Can you work these out from the model? Positions are in its coordinate system, mm. A direction names the side the tool comes from. Give positions to 0.01 mm unless a question says otherwise; leave off trailing zeros. Order: outer loops, then holes, each group sorted by start corner. A loop starts at its lowest first (then second) coordinate and runs counter-clockwise, first axis right, second up. Notation, with made-up numbers: M -5,-15.75 L 48,-15.75 A24 cw 48,22.25 Z; hole C -32.75,58 d5. An arc over 180 degrees is marked long. One line per question, with ' | ' between items. Start each with the question number.
1) Thinking about a two-plate mould opening in Z: for faces 4 (the flat face through (31.4, 12.5, -8.2)), 5 (the cylindrical face through (181.574, 10.528, -7.396)), 6 (the flat face through (107.6, 11.5, -19.9)), 7 (the flat face through (109, 8.5, -4)), which applies, +Z half, -Z half, draft (parallel to the pull), parting line (faces both ways), or undercut?
2) I'm going to push flat-ended pins straight in: pin 1 Ø3 at (x, y) = (149.5, 12) entering from +Z; pin 2 Ø3.5 at (x, y) = (180.5, 17) entering from +Z; pin 3 Ø4.5 at (x, z) = (31.5, -7.5) entering from +Y; pin 4 Ø2 at (x, z) = (180, -6.9) entering from +Y. Where does each tip first touch, or does it pass through?
3) For faces 1 (the flat face through (180, 16, -9.8)), 2 (the cylindrical face through (28.69, 10.53, -5.9)), 3 (the flat face through (107, 18.5, -12)), which set-ups out of +Z, -Z, +X, -X, +Y, -Y let a thin tool reach every point of the face, with its end or its side?
4) If we section it at B-B, the plane z = -14: Please give me the cut outline in (x, y).
5) Please list where these lines run through material, in increasing order: line 1 along X through (y, z) = (9.65, -6.9); line 2 along X through (y, z) = (10.6, -6.9); line 3 along X through (y, z) = (14.5, -15). Write a range as [from, to].
6) If we section it at A-A, the plane x = 23.5: Please give me the cut outline in (y, z), plus the area to 3 significant figures.
Autodesk Inventor part; units mm, degrees
ref_plane "YZ Plane" through (0, 0, 0) normal (1, 0, 0) x (0, 1, 0)
ref_plane "XZ Plane" through (0, 0, 0) normal (0, 1, 0) x (-1, 0, 0)
ref_plane "XY Plane" through (0, 0, 0) normal (0, 0, 1) x (1, 0, 0)
sketch "Sketch1" plane through (0, 0, 0) normal (1, 0, 0) x (0, 1, 0)
  circle A0 centre (0, 0) radius 20
  line L0 (8.5, 8.5) -> (-16.9, 8.5)
  line L1 (8.5, 8.5) -> (8.5, -16.9)
  line L2 (0, 0) -> (0, 20)
  line L3 (0, 20) -> (-60.9241, 20)
  line L4 (-60.9241, 20) -> (-60.9241, 18.5)
  line L5 (-60.9241, 18.5) -> (0, 18.5)
  line L6 (0, 18.5) -> (0, 20)
  line L7 (0, 0) -> (14.1421, 14.1421)
  line L8 (0, 0) -> (20, 0)
  line L9 (-16.9, 8.5) -> (-16.9, 18.5)
  line L10 (-16.9, 8.5) -> (-22.9, 14.5)
  line L11 (-22.9, 14.5) -> (-22.9, 18.5)
  line L12 (12.3744, 12.3744) -> (12.1502, 13.2109)
  line L13 (11.3137, 13.435) -> (9.2071, 11.3284)
  line L14 (9.4313, 10.4919) -> (10.2678, 10.2678)
  line L15 (8.5, 8.5) -> (8.5, -16.9)
  line L16 (20, 0) -> (20, -60.9241)
  line L17 (20, -60.9241) -> (18.5, -60.9241)
  line L18 (18.5, -60.9241) -> (18.5, 0)
  line L19 (8.5, -16.9) -> (18.5, -16.9)
  line L20 (8.5, -16.9) -> (14.5, -22.9)
  line L21 (14.5, -22.9) -> (18.5, -22.9)
  arc A1 (9.2071, 11.3284) -> (9.4313, 10.4919) centre (9.5607, 10.9749) ccw
  arc A2 (12.1502, 13.2109) -> (11.3137, 13.435) centre (11.6673, 13.0815) ccw
  line L22 (10.4311, 10.4311) -> (9.483, 10.6851)
  arc A3 (9.3485, 11.187) -> (9.483, 10.6851) centre (9.5607, 10.9749) ccw
  line L23 (9.3485, 11.187) -> (11.4551, 13.2936)
  arc A4 (11.957, 13.1591) -> (11.4551, 13.2936) centre (11.6673, 13.0815) ccw
  line L24 (11.957, 13.1591) -> (12.2111, 12.2111)
  point P0 (0, 8.5)
  point P1 (-17.7041, 9.3041)
  point P2 (-16.9, 10.6953)
  point P3 (10.6953, -16.9)
  point P4 (9.3041, -17.7041)
  point P5 (18.5, 0)
  dimension "d0" = 40
  dimension "d1" = 25.4
  dimension "d2" = 1.5
  dimension "d4" = 45
  dimension "d6" = 45
  dimension "d7" = 4
  dimension "d8" = 10
  dimension "d10" = 2.5
  dimension "d11" = 2.5
  dimension "d12" = 60
  dimension "d13" = 1.5
  dimension "d15" = 0.5
  dimension "d16" = 0.2
extrude "Extrusion1" add sketch "Sketch1" along normal blind 216 contours L8 L1 L7 A0 | L18 L19 A0 | A0 L19 L1 L8 L18 | L19 L18 L21 L20 A0 | A0 L20 L19
sketch "Sketch3" plane through (0, 18.5, 0) normal (0, 1, 0) x (1, 0, 0)
  line L0 (0, 22.9) -> (0, 0)
  line L1 (0, 0) -> (216, 0)
  line L2 (216, 22.9) -> (216, 0)
  line L3 (0, 22.9) -> (216, 22.9)
  line L4 (0, 16.9) -> (216, 16.9)
  line L5 (28.3257, 4) -> (26.6514, 6.9)
  line L6 (26.6514, 6.9) -> (28.3257, 9.8)
  line L7 (28.3257, 9.8) -> (31.6743, 9.8)
  line L8 (31.6743, 9.8) -> (33.3486, 6.9)
  line L9 (33.3486, 6.9) -> (31.6743, 4)
  line L10 (31.6743, 4) -> (28.3257, 4)
  circle A0 centre (30, 6.9) radius 1.65
  point P0 (0, 0)
  dimension "d28" = 5.8
  dimension "d29" = 10
  dimension "d30" = 30
  dimension "d31" = 3.3
extrude "Extrusion4" cut sketch "Sketch3" against normal blind 6 contours L5 L6 L7 L8 L9 L10 | A0
extrude "Extrusion5" cut sketch "Sketch3" against normal through all contours A0
sketch "Sketch4" plane through (0, 14.5, -22.9) normal (0, 0, -1) x (-1, 0, 0)
  line L0 (0, -6) -> (0, 0)
  line L1 (0, 0) -> (0, 4)
  line L2 (0, 4) -> (0, 5.5)
  line L3 (0, -6) -> (-216, -6)
  line L4 (0, 5.5) -> (-216, 5.5)
  line L5 (0, 5.5) -> (-4.787, -6)
  point P0 (0, -14.5)
  dimension "d36" = 112.6
extrude "Extrusion6" cut sketch "Sketch4" along normal through all both and the other way through all
pattern_linear "Rectangular Pattern1" count 2 spacing 150 along (1, 0, 0) of "Extrusion5", "Extrusion4"
sketch "Sketch5" plane through (2.4384, 14.1421, 14.1421) normal (0, -0.7071, 0.7071) x (1, 0, 0)
  line L0 (0, 0) -> (2.3486, -7.9792)
  line L1 (2.3486, -7.9792) -> (213.5616, -7.9792)
  line L2 (213.5616, 0) -> (213.5616, -7.9792)
  line L3 (0, 0) -> (213.5616, 0)
  circle A0 centre (193.5616, -4) radius 1.5
  line L4 (0, 0) -> (213.5616, 0)
  circle A1 centre (103.5616, -4) radius 1.5
  circle A2 centre (13.5616, -4) radius 1.5
  point P0 (-2.4384, -20)
  point P1 (106.7808, 0)
  point P2 (106.7808, 0)
  dimension "d42" = 3
  dimension "d44" = 4
  dimension "d45" = 20
  dimension "d48" = 90
extrude "Extrusion7" cut sketch "Sketch5" against normal blind 3 contours A0 | A1 | A2
properties part number "ESQUINA_REDONDEADA_R20" material "Steel, Mild, Welded"
Results found:
1) face 4: undercut | face 5: undercut | face 6: -Z half | face 7: draft
2) pin 1: stops at z = 13.5 | pin 2: stops at z = 12.94 | pin 3: stops at y = 18.5 | pin 4: passes through
3) face 1: +Y | face 2: +Y, -Y | face 3: -Z, +X, -X, +Y
4) outline: M 0.62,18.5 L 4.79,8.5 L 216,8.5 L 216,18.5 Z
5) line 1: x = [4.31, 28.35], [31.65, 178.35], [181.65, 216] | line 2: x = [3.91, 28.35], [31.65, 178.35], [181.65, 216] | line 3: x = [2.29, 216]
6) outline: M 8.5,-16.9 L 14.5,-22.9 L 18.5,-22.9 L 18.5,0 L 20,0 A20 ccw 14.14,14.14 L 8.5,8.5 Z | area: 332 mm²
